from build123d import *

# Parameters (mm, degrees)
FILLET1_R = 1


with BuildPart() as part:
    # Sketch1 → Revolve1 (revolve)
    with BuildSketch(Plane(origin=(0, 0, 0), x_dir=(1, 0, 0), z_dir=(0, 1, 0)), mode=Mode.PRIVATE) as revolve1_sk:
        Polygon((0, 7), (15, 7), (15, 8), (17, 8), (17, 5), (-2, 5), (-2, 8), (0, 8), align=None)
    revolve(revolve1_sk.sketch.rotate(Axis((0, 0, 0), (1, 0, 0)), 180), axis=Axis((0, 0, 0), (1, 0, 0)))

    # Fillet1
    fillet1_edges = [part.edges().sort_by_distance(p)[0] for p in [
        (0, 0, -7),
        (15, 0, -7),
    ]]
    fillet(fillet1_edges, radius=FILLET1_R - 0.0001)  # a hair under: the kernel refuses the full size


solid = part.part
The listing builds one solid part. Answer for the finished solid, in the listing's coordinates (mm). Coordinates: 2 decimals unless noted, no trailing zeros. Write each loop counter-clockwise with the first axis right and the second up, starting at its lowest first coordinate (ties: lowest second). Pieces come first, ordered by that corner, then holes. Notation, with made-up numbers: (11.25, 31) - (33.25, 31) arc R13 ccw to (33.25, 41) - close; hole circle Ø4 at (-3.5, -12). An arc over 180 degrees is marked (long way). Return JSON: item names as keys, results as strings.
1. For a pull along X with two mould halves and no side action, classify faces 1 (the face through (7.591, 2.681, 6.466)), 2 (the face through (16.01, 7.81, -1.73)), 3 (the face through (-2, 5.2, 0.1)) as +X half, -X half, draft (parallel to the pull), parting line (faces both ways), or undercut.
Final values:
{"face 1": "undercut", "face 2": "draft", "face 3": "-X half"}
2. Consider line 1 along Y through (x, z) = (2.5, 0); line 2 along Z through (x, y) = (13.5, -2.5); line 3 along Y through (x, z) = (8.5, 4.5). Determine where each line is inside the solid, lowest interval first.
Final values:
{"line 1": "-7 to -5, 5 to 7", "line 2": "-6.54 to -4.33, 4.33 to 6.54", "line 3": "-5.36 to -2.18, 2.18 to 5.36"}
3. The part is cut by section D-D on x = 15.75. Determine the outline of the cut face in (y, z).
Final values:
{"outline": "circle Ø16 at (0, 0); hole circle Ø10 at (0, 0)"}
4. The part is cut by section C-C on x = 4.25. Determine the outline of the cut face in (y, z).
Final values:
{"outline": "circle Ø14 at (0, 0); hole circle Ø10 at (0, 0)"}
5. Each of these flat-tipped pins is pushed along its axis until it touches: pin 1 Ø4 at (x, y) = (8, -1.5) entering from -Z; pin 2 Ø1 at (x, z) = (6, -4) entering from -Y; pin 3 Ø6 at (y, z) = (-1, -1.5) entering from +X; pin 4 Ø8 at (x, y) = (7.5, 6) entering from -Z. Where does it stop, or does it pass through?
Final values:
{"pin 1": "z = -7", "pin 2": "y = -6.06", "pin 3": "through", "pin 4": "z = -6.71"}
